```python
from build123d import *

# Parameters (mm, degrees)
SKETCH1_W           = 11
SKETCH1_H           = 9
BOSS_EXTRUDE1_DEPTH = 3.175
BOSS_EXTRUDE2_DEPTH = 3.175
SKETCH3_W           = 27.735440415
SKETCH3_H           = 29.716543301
BOSS_EXTRUDE3_DEPTH = 3.175
SKETCH4_R           = 3.175
CUT_EXTRUDE1_DEPTH  = 3.175


with BuildPart() as part:
    # Sketch1 → Boss-Extrude1 (new body)
    with BuildSketch(Plane(origin=(0, 0, 0), x_dir=(1, 0, 0), z_dir=(0, 1, 0))):
        Polygon((-68.253472382, 16.682663469), (-68.253472382, -31.317336531), (57.746527618, -31.317336531), (57.746527618, -18.067336531), (35.746527618, -18.067336531), (35.746527618, 5.932663469), (57.746527618, 5.932663469), (57.746527618, 16.682663469), (-21.910593359, 16.682663469), (-21.910593359, 3.082663469), (-24.310593359, 0.682663469), (-27.510593359, 0.682663469), (-29.910593359, 3.082663469), (-29.910593359, 16.682663469), (-36.877993049, 16.682663469), (-36.877993049, -5.317336531), (-53.877993049, -5.317336531), (-53.877993049, 16.682663469), align=None)
        with Locations((-25.910593359, -9.817336531)):
            Rectangle(SKETCH1_W, SKETCH1_H, mode=Mode.SUBTRACT)
    extrude(amount=BOSS_EXTRUDE1_DEPTH)

    # Sketch2 → Boss-Extrude2 (add)
    with BuildSketch(Plane(origin=(0, 3.175, 0), x_dir=(1, 0, 0), z_dir=(0, 1, 0))):
        Polygon((59.746527618, 16.682663469), (57.746527618, 16.682663469), (57.746527618, 5.932663469), (57.746527618, -18.067336531), (57.746527618, -31.317336531), (-68.253472382, -31.317336531), (-68.253472382, -33.317336531), (59.746527618, -33.317336531), align=None)
    extrude(amount=-BOSS_EXTRUDE2_DEPTH)

    # Sketch3 → Boss-Extrude3 (add)
    with BuildSketch(Plane(origin=(0, 3.175, 0), x_dir=(1, 0, 0), z_dir=(0, 1, 0))):
        with Locations((44.64848835, -4.824339336)):
            Rectangle(SKETCH3_W, SKETCH3_H)
    extrude(amount=-BOSS_EXTRUDE3_DEPTH)

    # Sketch4 → Cut-Extrude1 (cut)
    with BuildSketch(Plane(origin=(0, 3.175, 0), x_dir=(1, 0, 0), z_dir=(0, 1, 0))):
        with Locations((-8.479841083, 5.611362845)):
            Circle(SKETCH4_R)
        with Locations((3.520158917, 5.611362845)):
            Circle(SKETCH4_R)
        with Locations((15.520158917, 5.611362845)):
            Circle(SKETCH4_R)
        with Locations((27.520158917, 5.611362845)):
            Circle(SKETCH4_R)
        with Locations((39.520158917, 5.611362845)):
            Circle(SKETCH4_R)
        with Locations((51.520158917, 5.611362845)):
            Circle(SKETCH4_R)
        with Locations((-14.20477293, -2.36159985)):
            Circle(SKETCH4_R)
        with Locations((-2.20477293, -2.36159985)):
            Circle(SKETCH4_R)
        with Locations((9.79522707, -2.36159985)):
            Circle(SKETCH4_R)
        with Locations((21.79522707, -2.36159985)):
            Circle(SKETCH4_R)
        with Locations((33.79522707, -2.36159985)):
            Circle(SKETCH4_R)
        with Locations((45.79522707, -2.36159985)):
            Circle(SKETCH4_R)
        with Locations((-8.244355205, -10.556666731)):
            Circle(SKETCH4_R)
        with Locations((3.755644795, -10.556666731)):
            Circle(SKETCH4_R)
        with Locations((15.755644795, -10.556666731)):
            Circle(SKETCH4_R)
        with Locations((27.755644795, -10.556666731)):
            Circle(SKETCH4_R)
        with Locations((39.755644795, -10.556666731)):
            Circle(SKETCH4_R)
        with Locations((51.755644795, -10.556666731)):
            Circle(SKETCH4_R)
        with Locations((-13.969287051, -18.529629426)):
            Circle(SKETCH4_R)
        with Locations((-1.969287051, -18.529629426)):
            Circle(SKETCH4_R)
        with Locations((10.030712949, -18.529629426)):
            Circle(SKETCH4_R)
        with Locations((22.030712949, -18.529629426)):
            Circle(SKETCH4_R)
        with Locations((34.030712949, -18.529629426)):
            Circle(SKETCH4_R)
        with Locations((46.030712949, -18.529629426)):
            Circle(SKETCH4_R)
    extrude(amount=-CUT_EXTRUDE1_DEPTH, mode=Mode.SUBTRACT)


solid = part.part
```
Part model, mm, in its own coordinate system. A direction names the side the tool comes from. Give positions to 0.01 mm unless a question says otherwise; leave off trailing zeros. Write each loop counter-clockwise with the first axis right and the second up, starting at its lowest first coordinate (ties: lowest second). Pieces come first, ordered by that corner, then holes. Notation, with made-up numbers: M 20.5,47 L 33.5,47 A27 ccw 33.5,75 Z; hole C 29,72 d5. An arc over 180 degrees is marked long. Use CSV: the item, a comma, the result in double quotes.
Item 1: Slice it at B-B on x = -7. Write the cut outline in (y, z) (3 decimals).
Taken from the geometry:
outline,"M 0,-16.683 L 3.175,-16.683 L 3.175,-8.42 L 0,-8.42 Z; M 0,-2.802 L 3.175,-2.802 L 3.175,7.636 L 0,7.636 Z; M 0,13.478 L 3.175,13.478 L 3.175,33.317 L 0,33.317 Z"
Item 2: Which spindle directions (+Z, -Z, +X, -X, +Y, -Y) get a long thin tool onto all of the face, cutting with end or side? Do faces 5 (the face through (-5, 3.175, 8)), 6 (the face through (-53.878, 2, -6)), 7 (the face through (-26, 2, 14.317)). Say none if no direction does.
Taken from the geometry:
face 5,"+Z, -Z, +X, -X, +Y"
face 6,"-Z, +Y, -Y"
face 7,"+Y, -Y"
Item 3: Slice it at C-C on x = -47. Write the cut outline in (y, z) (3 decimals).
Taken from the geometry:
outline,"M 0,5.317 L 3.175,5.317 L 3.175,33.317 L 0,33.317 Z"
Item 4: Pin check, flat tip, straight feed: P1, Ø1.6, axis at x = -42, y = 2.5, coming from the -Z side. Stop position of the tip, or through.
Taken from the geometry:
P1,"stops at z = 5.32"
Item 5: Pull direction X, two halves, no side cores. Call faces 1 (the face through (36.584, 1.61, 10.417)), 2 (the face through (-26, 2, 5.317)), 3 (the face through (-33, 2, -16.683)), 4 (the face through (59.747, 2, 9)): +X half, -X half, draft (parallel to the pull), parting line (faces both ways), or undercut.
Taken from the geometry:
face 1,"undercut"
face 2,"undercut"
face 3,"draft"
face 4,"+X half"
Item 6: Slice it at A-A on z = -12. Write the cut outline in (x, y) (3 decimals), plus the area to 3 significant figures.
Taken from the geometry:
outline,"M -68.253,0 L -53.878,0 L -53.878,3.175 L -68.253,3.175 Z; M -36.878,0 L -29.911,0 L -29.911,3.175 L -36.878,3.175 Z; M -21.911,0 L 59.747,0 L 59.747,3.175 L -21.911,3.175 Z"
area,"327 mm²"
Item 7: Slice it at D-D on y = 0.95. State how many separate pieces and enclosed holes the cut face has, plus the area to 3 significant figures.
Taken from the geometry:
separate pieces,"1"
enclosed holes,"25"
area,"5,040 mm²"
Item 8: Drill centre lines: probe 1 along Z at (x, y) = (-31, 1.55); probe 2 along Z at (x, y) = (13.5, 2.4); probe 3 along Z at (x, y) = (-47.5, 0.35). Where is each one in solid material? Low to high.
Taken from the geometry:
probe 1,"z = -16.68 to 5.32, 14.32 to 33.32"
probe 2,"z = -16.68 to -8.06, -3.16 to 8.32, 12.79 to 33.32"
probe 3,"z = 5.32 to 33.32"
